```python
from build123d import *

# Parameters (mm, degrees)
SKETCH1_W           = 90
SKETCH1_H           = 42
SKETCH1_W_2         = 14
SKETCH1_H_2         = 14
SKETCH1_H_3         = 20
SKETCH1_W_3         = 8
SKETCH1_H_4         = 8
BOSS_EXTRUDE1_DEPTH = 3
FILLET1_R           = 5
FILLET2_R           = 2
SKETCH3_R           = 1.25
CUT_EXTRUDE1_DEPTH  = 3
SKETCH4_R           = 1.25
CUT_EXTRUDE2_DEPTH  = 3


with BuildPart() as part:
    # Sketch1 → Boss-Extrude1 (new body)
    with BuildSketch(Plane.XY):
        Rectangle(SKETCH1_W, SKETCH1_H)
        with Locations((-45, 21)):
            Rectangle(SKETCH1_W_2, SKETCH1_H_2)
        with Locations((45, 21)):
            Rectangle(SKETCH1_W_2, SKETCH1_H_2)
        with Locations((45, -21)):
            Rectangle(SKETCH1_W_2, SKETCH1_H_2)
        with Locations((-45, -21)):
            Rectangle(SKETCH1_W_2, SKETCH1_H_2)
        with Locations((0, 21)):
            Rectangle(SKETCH1_W_2, SKETCH1_H_3)
        with Locations((0, -21)):
            Rectangle(SKETCH1_W_2, SKETCH1_H_3)
        with Locations((30, 21)):
            Rectangle(SKETCH1_W_3, SKETCH1_H_4)
        with Locations((-30, 21)):
            Rectangle(SKETCH1_W_3, SKETCH1_H_4)
        with Locations((30, -21)):
            Rectangle(SKETCH1_W_3, SKETCH1_H_4)
        with Locations((-30, -21)):
            Rectangle(SKETCH1_W_3, SKETCH1_H_4)
    extrude(amount=BOSS_EXTRUDE1_DEPTH)

    # Fillet1
    fillet1_edges = [part.edges().sort_by_distance(p)[0] for p in [
        (52, 14, 1.5),
        (52, 28, 1.5),
        (38, 28, 1.5),
        (7, 31, 1.5),
        (-7, 31, 1.5),
        (-38, 28, 1.5),
        (-52, 28, 1.5),
        (-52, 14, 1.5),
        (-52, -14, 1.5),
        (-52, -28, 1.5),
        (-38, -28, 1.5),
        (-7, -31, 1.5),
        (7, -31, 1.5),
        (38, -28, 1.5),
        (52, -28, 1.5),
        (52, -14, 1.5),
    ]]
    fillet(fillet1_edges, radius=FILLET1_R)

    # Fillet2
    fillet2_edges = [part.edges().sort_by_distance(p)[0] for p in [
        (-26, 25, 1.5),
        (-26, 21, 1.5),
        (-34, 25, 1.5),
        (-34, 21, 1.5),
        (-38, 21, 1.5),
        (34, 21, 1.5),
        (7, 21, 1.5),
        (26, 25, 1.5),
        (34, 25, 1.5),
        (38, 21, 1.5),
        (26, 21, 1.5),
        (-7, 21, 1.5),
        (45, 14, 1.5),
        (45, -14, 1.5),
        (38, -21, 1.5),
        (34, -21, 1.5),
        (34, -25, 1.5),
        (26, -25, 1.5),
        (26, -21, 1.5),
        (-7, -21, 1.5),
        (7, -21, 1.5),
        (-26, -21, 1.5),
        (-26, -25, 1.5),
        (-34, -25, 1.5),
        (-34, -21, 1.5),
        (-38, -21, 1.5),
        (-45, -14, 1.5),
        (-45, 14, 1.5),
    ]]
    fillet(fillet2_edges, radius=FILLET2_R - 0.0001)  # a hair under: the kernel refuses the full size

    # Sketch3 → Cut-Extrude1 (cut)
    with BuildSketch(Plane.XY.offset(3)):
        with Locations((-30, 21)):
            Circle(SKETCH3_R)
        with Locations((30, 21)):
            Circle(SKETCH3_R)
        with Locations((30, -21)):
            Circle(SKETCH3_R)
        with Locations((-30, -21)):
            Circle(SKETCH3_R)
    extrude(amount=-CUT_EXTRUDE1_DEPTH, mode=Mode.SUBTRACT)

    # Sketch4 → Cut-Extrude2 (cut)
    with BuildSketch(Plane.XY.offset(3)):
        with Locations((35, 0)):
            Circle(SKETCH4_R)
    extrude(amount=-CUT_EXTRUDE2_DEPTH, mode=Mode.SUBTRACT)


solid = part.part
```
Read the model definition and answer for the solid it produces. Units are mm, in the model's axes. A direction names the side the tool comes from. Coordinates: 2 decimals unless noted, no trailing zeros. Write each loop counter-clockwise with the first axis right and the second up, starting at its lowest first coordinate (ties: lowest second). Pieces come first, ordered by that corner, then holes. Notation, with made-up numbers: (61, -12) -> (102, -12) arc R19 cw to (102, 20) -> close; hole circle Ø4 at (36.25, -17). An arc over 180 degrees is marked (long way). Answer as a JSON object with one key per item and string values.
Q1. Determine the mould class of faces 1 (the cylindrical face through (45.6, -13.43, 1.52)), 2 (the flat face through (0, 31, 1)), 3 (the flat face through (45, -28, 1)) for opening direction Y: pulls with the +Y half, pulls with the -Y half, needs draft (parallel to the pull), parting line crosses it, or undercut.
The answers:
{"face 1": "undercut", "face 2": "pulls with the +Y half", "face 3": "pulls with the -Y half"}
Q2. Flat-ended cylindrical pins translate along their axes: pin 1 Ø0.9 at (y, z) = (-2, 2) entering from -X; pin 2 Ø1.5 at (x, z) = (-30, 1.5) entering from -Y; pin 3 Ø2 at (x, y) = (-30, -21) entering from -Z; pin 4 Ø0.9 at (x, z) = (-29.5, 1.5) entering from +Y. Find the tip coordinate at first contact, or state that the pin passes through.
The answers:
{"pin 1": "stops at x = -45", "pin 2": "stops at y = -25", "pin 3": "passes through", "pin 4": "stops at y = 25"}
Q3. The part is cut by section D-D on x = 39. Give the vertices of the cut face in (y, z).
The answers:
{"outline": "(-26, 0) -> (26, 0) -> (26, 3) -> (-26, 3) -> close"}
Q4. A tool of negligible diameter and unlimited length cuts with its end or side. For faces 4 (the cylindrical face through (-40, -27, 2)), 5 (the cylindrical face through (40, 27, 2)), 6 (the cylindrical face through (50, 15, 2)), 7 (the flat face through (-45, -28, 1)), 8 (the cylindrical face through (-51, 16, 2)), from which of +Z, -Z, +X, -X, +Y, -Y can it reach the whole face along a straight path? Write none if from no direction.
The answers:
{"face 4": "+Z, -Z, -Y", "face 5": "+Z, -Z, +Y", "face 6": "+Z, -Z, +X", "face 7": "+Z, -Z, -X, -Y", "face 8": "+Z, -Z, -X"}
Q5. The part is cut by section B-B on y = 0. Give the vertices of the cut face in (x, z).
The answers:
{"outline": "(-45, 0) -> (33.75, 0) -> (33.75, 3) -> (-45, 3) -> close; (36.25, 0) -> (45, 0) -> (45, 3) -> (36.25, 3) -> close"}
Q6. The part is cut by section C-C on z = 1.45. Give the number of separate pieces and of enclosed holes in the cut face, then the cut area to 3 significant figures.
The answers:
{"separate pieces": "1", "enclosed holes": "5", "area": "4,680 mm2"}
Q7. The part is cut by section A-A on x = -30. Give the vertices of the cut face in (y, z), then the cut area to 3 significant figures.
The answers:
{"outline": "(-25, 0) -> (-22.25, 0) -> (-22.25, 3) -> (-25, 3) -> close; (-19.75, 0) -> (19.75, 0) -> (19.75, 3) -> (-19.75, 3) -> close; (22.25, 0) -> (25, 0) -> (25, 3) -> (22.25, 3) -> close", "area": "135 mm2"}
Q8. Consider line 1 (Y direction, x = 30, z = 0.8); line 2 (Y direction, x = -29.5, z = 0.75); line 3 (X direction, y = -23.5, z = 0.7). Determine where each line is inside the solid, lowest interval first. Write a range as [from, to].
The answers:
{"line 1": "y = [-25, -22.25], [-19.75, 19.75], [22.25, 25]", "line 2": "y = [-25, -22.15], [-19.85, 19.85], [22.15, 25]", "line 3": "x = [-51.97, -38.03], [-33.94, -26.06], [-7, 7], [26.06, 33.94], [38.03, 51.97]"}
